Part model, mm, in its own coordinate system. A direction names the side the tool comes from. Coordinates: 2 decimals unless noted, no trailing zeros. Loops run counter-clockwise (first coordinate to the right, second up) from the corner with the lowest first, then second, coordinate; pieces in that order, holes last. Notation, with made-up numbers: (58, 20) -> (73, 20) arc R24 ccw to (73, 36) -> close; hole circle Ø5 at (-40, 20.5). An arc over 180 degrees is marked (long way). Use one line per item in the form item = value. Start each with the question number.
(1) Drill centre lines: L1, parallel to Z at x = 128.5, y = 71; L2, parallel to Z at x = -89, y = 47; L3, parallel to Y at x = 94, z = 108.5. Where is each one in solid material? Low to high. Write a range as [from, to].
(2) Pin check, flat tips, straight feed: P1, Ø13, axis at x = -122.5, y = 46.5, coming from the +Z side; P2, Ø7.5, axis at x = -129.5, y = 78, coming from the -Z side; P3, Ø3, axis at x = 86.5, y = -37, coming from the +Z side; P4, Ø20, axis at x = 107.5, z = 121, coming from the +Y side. Stop position of each tip, or through.
(3) Mould opens along X. For faces 4 (the flat face through (-2, 1, 0)), 5 (the cylindrical face through (93.51, 27.58, 129.15)), 6 (the flat face through (-140.1, -82.4, 39.4)) say: +X half, -X half, draft (parallel to the pull), parting line (faces both ways), or undercut.
(4) Band-saw the part on A-A on x = -105. Give the cut face in (y, z), then the cut area to 3 significant figures.
(5) Band-saw the part on C-C on x = -17. Give the cut face in (y, z), then the cut area to 3 significant figures.
(6) 3-axis set-ups, long thin cutter, end or side, ignore diameter. For faces 1 (the flat face through (-132.3, 75.2, 39.4)), 2 (the flat face through (130, 78, 80)), 3 (the flat face through (133.5, 41, 91)): which of +Z, -Z, +X, -X, +Y, -Y reach the whole face in a straight line?
(7) Band-saw the part on B-B on y = -50.5. Give the cut face in (x, z).
```python
from build123d import *

# Parameters (mm, degrees)
EXTRUDE_1_DEPTH = 80
SKETCH_2_W      = 43
SKETCH_2_H      = 60
EXTRUDE_2_DEPTH = 12
SKETCH_3_W      = 43
SKETCH_3_H      = 12
EXTRUDE_3_DEPTH = 40
FILLET_1_R      = 10


with BuildPart() as part:
    # 草图1 → 凸台-拉伸1 (new body)
    with BuildSketch(Plane.XY):
        Polygon((-145, -77.5), (-135, -87.5), (135, -87.5), (145, -77.5), (145, 62.5), (120, 87.5), (-120, 87.5), (-145, 62.5), align=None)
    extrude(amount=EXTRUDE_1_DEPTH)

    # 草图2 → 凸台-拉伸2 (add)
    with BuildSketch(Plane.XY.offset(80)):
        with Locations((-112, 51.5)):
            Rectangle(SKETCH_2_W, SKETCH_2_H)
        with Locations((112, 51.5)):
            Rectangle(SKETCH_2_W, SKETCH_2_H)
    extrude(amount=EXTRUDE_2_DEPTH)

    # 草图3 → 凸台-拉伸3 (add)
    with BuildSketch(Plane.XY.offset(92)):
        with Locations((-112, 27.5)):
            Rectangle(SKETCH_3_W, SKETCH_3_H)
        with Locations((112, 27.5)):
            Rectangle(SKETCH_3_W, SKETCH_3_H)
    extrude(amount=EXTRUDE_3_DEPTH)

    # 圆角1
    # the kernel refuses this fillet: 10 mm, written as the material it takes off along each edge
    with BuildSketch(Plane(origin=(-90.5, 81.5, 80), x_dir=(-1, 0, 0), z_dir=(0, 0, 1)), Plane(origin=(90.5, 81.5, 80), x_dir=(0, -1, 0), z_dir=(0, 0, 1))) as fillet_1_piece_1:
        with BuildLine():
            CenterArc((FILLET_1_R, FILLET_1_R), FILLET_1_R, 180, 90)
            Line((0, FILLET_1_R), (0, 0))
            Line((0, 0), (FILLET_1_R, 0))
        make_face()
    extrude(amount=37, mode=Mode.SUBTRACT)
    with BuildSketch(Plane(origin=(-133.5, 81.5, 80), x_dir=(1, 0, 0), z_dir=(0, 0, 1)), Plane(origin=(133.5, 81.5, 80), x_dir=(0, -1, 0), z_dir=(0, 0, 1))) as fillet_1_piece_2:
        with BuildLine():
            CenterArc((FILLET_1_R, -FILLET_1_R), FILLET_1_R, 90, 90)
            Line((0, -FILLET_1_R), (0, 0))
            Line((0, 0), (FILLET_1_R, 0))
        make_face()
    extrude(amount=37, mode=Mode.SUBTRACT)
    with BuildSketch(Plane(origin=(-133.5, 58.5, 132), x_dir=(1, 0, 0), z_dir=(0, -1, 0)), Plane(origin=(-90.5, -3.5, 132), x_dir=(-1, 0, 0), z_dir=(0, 1, 0)), Plane(origin=(90.5, 58.5, 132), x_dir=(1, 0, 0), z_dir=(0, -1, 0))) as fillet_1_piece_3:
        with BuildLine():
            CenterArc((FILLET_1_R, -FILLET_1_R), FILLET_1_R, 90, 90)
            Line((0, -FILLET_1_R), (0, 0))
            Line((0, 0), (FILLET_1_R, 0))
        make_face()
    extrude(amount=62, mode=Mode.SUBTRACT)
    with BuildSketch(Plane(origin=(133.5, -3.5, 132), x_dir=(0, 0, -1), z_dir=(0, 1, 0))) as fillet_1_piece_4:
        with BuildLine():
            CenterArc((FILLET_1_R, FILLET_1_R), FILLET_1_R, 180, 90)
            Line((0, FILLET_1_R), (0, 0))
            Line((0, 0), (FILLET_1_R, 0))
        make_face()
    extrude(amount=62, mode=Mode.SUBTRACT)


solid = part.part
```
A:
q1.L1 = [0, 92]
q1.L2 = [0, 80]
q1.L3 = [21.5, 33.5]
q2.P1 = 92
q2.P2 = 0
q2.P3 = 80
q2.P4 = 33.5
q3.face_4 = draft
q3.face_5 = undercut
q3.face_6 = -X half
q4.outline = (-87.5, 0) -> (87.5, 0) -> (87.5, 80) -> (81.5, 80) -> (81.5, 92) -> (33.5, 92) -> (33.5, 132) -> (21.5, 132) -> (21.5, 80) -> (-87.5, 80) -> close
q4.area = 15,200 mm²
q5.outline = (-87.5, 0) -> (87.5, 0) -> (87.5, 80) -> (-87.5, 80) -> close
q5.area = 14,000 mm²
q6.face_1 = -Z, -X, +Y
q6.face_2 = -Z, +X, +Y
q6.face_3 = +Z, +X, +Y, -Y
q7.outline = (-145, 0) -> (145, 0) -> (145, 80) -> (-145, 80) -> close
